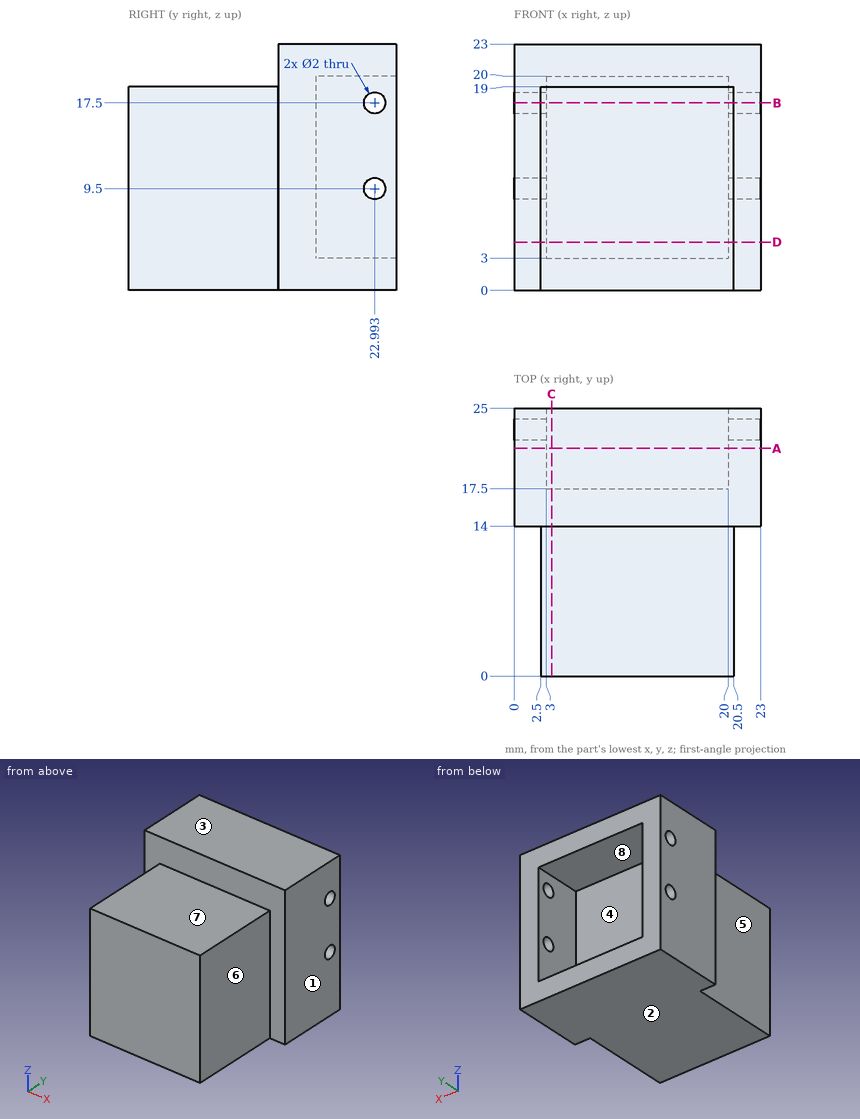
Design review of the part shown in the three views and the two pictorial views. Dimensions are in mm from the part's minimum x, y and z. A direction names the side the tool comes from. Coordinates: 2 decimals unless noted, no trailing zeros. Loops run counter-clockwise (first coordinate to the right, second up) from the corner with the lowest first, then second, coordinate; pieces in that order, holes last. Notation, with made-up numbers: M 50.5,56.25 L 95.5,56.25 A10 ccw 95.5,64.25 Z; hole C -12.75,42.5 d1. An arc over 180 degrees is marked long. Put each result on its own line as item: value. Start each with the question number.
Q1. Add section A-A (y = 21.25). Write out the cut boundary in (x, z), and give its area (3 significant figures).
Q2. Wall thickness on line 1 (Y direction, x = 1.7, z = 9.5); line 2 (X direction, y = 22, z = 16.75): over which ranges is each line inside the solid? List them lowest first.
Q3. Clearance check with flat-ended pins moving along their axes: pin 1 (4 mm diameter, centred on x = 17.5, z = 13, fed in from +Y); pin 2 (4 mm diameter, centred on y = 7, z = 6.5, fed in from -X); pin 3 (1.8 mm diameter, centred on y = 22.99, z = 17.5, fed in from -X); pin 4 (11 mm diameter, centred on y = 6, z = 8, fed in from +X). State where each tip first meets the part, or that it passes through.
Q4. For the marked faces 5, 6, 7 and 8, list the 3-axis set-ups (+Z, -Z, +X, -X, +Y, -Y) from which the entire face can be reached by the end or side of a thin tool; tool diameter is ignored.
Q5. The part is to be moulded in two halves that separate along Z. For the marked faces 1, 2, 3 and 4, say which applies: +Z half, -Z half, draft (parallel to the pull), parting line (faces both ways), or undercut.
Q6. Add section D-D (z = 4.5). Write out the cut boundary in (x, y), and give its area (4 significant figures).
Q7. Add section C-C (x = 3.5). Write out the cut boundary in (y, z), and give its area (4 significant figures).
Q8. Add section B-B (z = 17.5). Write out the cut boundary in (x, y).
Answers:
1. outline: M 0,0 L 23,0 L 23,23 L 0,23 Z; hole M 3,3 L 20,3 L 20,20 L 3,20 Z
1. area: 240 mm^2
2. line 1: y = 14 to 21.99, 23.99 to 25
2. line 2: x = 0 to 3, 20 to 23
3. pin 1: stops at y = 17.5
3. pin 2: stops at x = 2.5
3. pin 3: passes through
3. pin 4: stops at x = 20.5
4. face 5: +Z, -Z, -X, -Y
4. face 6: +Z, -Z, +X, -Y
4. face 7: +Z, +X, -X, -Y
4. face 8: +Y
5. face 1: draft
5. face 2: -Z half
5. face 3: +Z half
5. face 4: undercut
6. outline: M 0,14 L 2.5,14 L 2.5,0 L 20.5,0 L 20.5,14 L 23,14 L 23,25 L 20,25 L 20,17.5 L 3,17.5 L 3,25 L 0,25 Z
6. area: 377.5 mm^2
7. outline: M 0,0 L 25,0 L 25,3 L 17.5,3 L 17.5,20 L 25,20 L 25,23 L 14,23 L 14,19 L 0,19 Z
7. area: 391.5 mm^2
8. outline: M 0,14 L 2.5,14 L 2.5,0 L 20.5,0 L 20.5,14 L 23,14 L 23,21.99 L 20,21.99 L 20,17.5 L 3,17.5 L 3,21.99 L 0,21.99 Z; M 0,23.99 L 3,23.99 L 3,25 L 0,25 Z; M 20,23.99 L 23,23.99 L 23,25 L 20,25 Z
